Geometry check sheet. Reference: drawing and pictorial views, mm from the part's lowest x, y, z. Round coordinates to 2 decimals unless told otherwise and drop trailing zeros. Order: outer loops, then holes, each group sorted by start corner. A loop starts at its lowest first (then second) coordinate and runs counter-clockwise, first axis right, second up.
(1) Sectioned sample at C-C, the plane y = 1.25. Count the separate pieces of the cut face and the enclosed holes in it, and give its area (3 significant figures).
(2) Sectioned sample at B-B, the plane z = 2.5. Enter the section's corners in (x, y) (1 decimal).
(3) Depth check by flat-ended pin: pin 1 (1.2 mm diameter, centred on y = 4.5, z = 8.5, fed in from -X); pin 2 (11 mm diameter, centred on x = 6.35, z = 9.525, fed in from +Y) (1 decimal). Enter the tip coordinate at first touch or a pass-through.
(4) Thickness scan on probe 1 along Z at (x, y) = (76.2, 2.75); probe 2 along Z at (x, y) = (6.35, 1.1); probe 3 along X at (y, z) = (6.25, 2). Record the ranges inside material, lowest first.
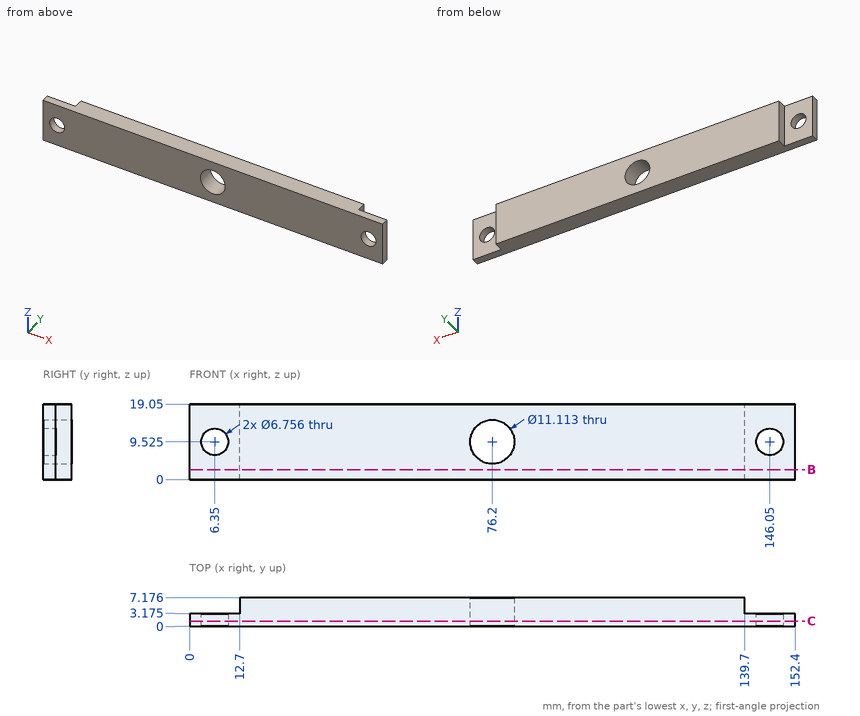
Derived:
1. separate pieces: 1
1. enclosed holes: 3
1. area: 2,730 mm2
2. outline: (0, 0) - (152.4, 0) - (152.4, 3.2) - (139.7, 3.2) - (139.7, 7.2) - (12.7, 7.2) - (12.7, 3.2) - (0, 3.2) - close
3. pin 1: stops at x = 12.7
3. pin 2: stops at y = 3.2
4. probe 1: z = 0 to 3.97, 15.08 to 19.05
4. probe 2: z = 0 to 6.15, 12.9 to 19.05
4. probe 3: x = 12.7 to 139.7
